```python
from build123d import *

# Parameters (mm, degrees)
SKETCH1_R           = 13.45
BOSS_EXTRUDE2_DEPTH = 48
SKETCH7_W           = 44
SKETCH7_H           = 14
SKETCH7_R           = 4.25
SKETCH7_R_2         = 4.1
BOSS_EXTRUDE3_DEPTH = 13
FILLET1_R           = 3
FILLET2_R           = 5
FILLET3_R           = 5
FILLET4_R           = 3


with BuildPart() as part:
    # Sketch1 → Boss-Extrude2 (new body)
    with BuildSketch(Plane(origin=(0, 0, 0), x_dir=(1, 0, 0), z_dir=(0, 1, 0))):
        Polygon((-17.4, 17.4), (17.4, 17.4), (17.4, -17.4), (-17.4, -17.4), (-17.4, 13.4), (-82.6, 13.4), (-82.6, 17.4), align=None)
        with Locations(Location((0, 0, 0), (0, 0, 270))):
            Circle(SKETCH1_R, mode=Mode.SUBTRACT)
    boss_extrude2 = extrude(amount=BOSS_EXTRUDE2_DEPTH)

    # Mirror2: Boss-Extrude2 across plane
    add(boss_extrude2.mirror(Plane(origin=(-82.6, 48, -17.4), x_dir=(0, 0, 1), z_dir=(1, 0, 0))))

    # Sketch7 → Boss-Extrude3 (add)
    with BuildSketch(Plane.XY.offset(-13.4)):
        with Locations((-97.6, 24)):
            Rectangle(SKETCH7_W, SKETCH7_H)
        with Locations(Location((-82.6, 24, 0), (0, 0, 180))):
            Circle(SKETCH7_R, mode=Mode.SUBTRACT)
        with Locations(Location((-112.6, 24, 0), (0, 0, 180))):
            Circle(SKETCH7_R_2, mode=Mode.SUBTRACT)
    extrude(amount=BOSS_EXTRUDE3_DEPTH)

    # Fillet1
    fillet1_edges = [part.edges().sort_by_distance(p)[0] for p in [
        (17.4, 24, 17.4),
        (-17.4, 24, 17.4),
        (-182.6, 24, 17.4),
        (-147.8, 24, 17.4),
    ]]
    fillet(fillet1_edges, radius=FILLET1_R)

    # Fillet2
    fillet2_edges = [part.edges().sort_by_distance(p)[0] for p in [
        (-17.4, 24, -13.4),
        (17.4, 24, -17.4),
        (-182.6, 24, -17.4),
        (-147.8, 24, -13.4),
    ]]
    fillet(fillet2_edges, radius=FILLET2_R)

    # Fillet3
    fillet3_edges = [part.edges().sort_by_distance(p)[0] for p in [
        (-75.6, 17, -6.9),
        (-75.6, 31, -6.9),
        (-119.6, 31, -6.9),
        (-119.6, 17, -6.9),
    ]]
    fillet(fillet3_edges, radius=FILLET3_R)

    # Fillet4
    fillet4_edges = [part.edges().sort_by_distance(p)[0] for p in [
        (-97.6, 31, -13.4),
        (-75.6, 24, -13.4),
        (-97.6, 17, -13.4),
        (-119.6, 24, -13.4),
        (-77.064466094, 29.535533906, -13.4),
        (-77.064466094, 18.464466094, -13.4),
        (-118.135533906, 29.535533906, -13.4),
        (-118.135533906, 18.464466094, -13.4),
    ]]
    fillet(fillet4_edges, radius=FILLET4_R)


solid = part.part
```
Geometry: final body of the model. Coordinates: model frame, mm. A direction names the side the tool comes from. Give positions to 0.01 mm unless a question says otherwise; leave off trailing zeros. Loops run counter-clockwise (first coordinate to the right, second up) from the corner with the lowest first, then second, coordinate; pieces in that order, holes last. Notation, with made-up numbers: (20, 75.5) - (66, 75.5) arc R23 cw to (66, 87.5) - close; hole circle Ø9 at (8.25, 5.5). An arc over 180 degrees is marked (long way). Answer as CSV lines item,"result". Start each with the question number.
(1) Reachability of faces 4 (the face through (-98, 31, -5)), 5 (the face through (-17.4, 24, 3)), 6 (the face through (-118.17, 18.5, -5.33)) from +Z, -Z, +X, -X, +Y, -Y: full face, straight path, thin tool, end or side. Return the list, or none.
(2) Pin query (flat end, axial travel): P1, Ø15.5, axis at x = -102.5, y = 25, coming from the +Z side; P2, Ø11, axis at x = -103.5, z = -3, coming from the +Y side; P3, Ø16, axis at x = -165.2, z = 0, coming from the +Y side; P4, Ø3, axis at y = 14.5, z = -13.5, coming from the -X side. Return the tip coordinate at first contact, or that it passes through.
(3) Ray query, line 1 along X through (y, z) = (22.5, 0); line 2 along Y through (x, z) = (-112.6, -5.25); line 3 along Y through (x, z) = (-82.6, -4.75). Return the intervals inside material, ascending. Write a range as [from, to].
(4) Mould query, pull axis X, two halves, no side actions, for faces 1 (the face through (-181.17, 24.34, -15.9)), 2 (the face through (-18.9, 24.34, -11.97)), 3 (the face through (-165, 24, 17.4)). Classes: +X half, -X half, draft (parallel to the pull), parting line (faces both ways), or undercut.
(5) Section query B-B (z = -3). Output: boundary loops of the cut face in (x, y).
(6) Section query C-C (y = 24). Give the number of separate pieces and of enclosed holes in the cut face, and give its area (3 significant figures).
(7) Section query D-D (z = 11.5). Output: boundary loops of the cut face in (x, y).
(8) Section query A-A (x = 0). Output: boundary loops of the cut face in (y, z), and give its area (3 significant figures).
Worked answers:
1,face 4,"+Z, +Y"
1,face 5,"+Z, +Y, -Y"
1,face 6,"+Z, -Y"
2,P1,"stops at z = -0.4"
2,P2,"stops at y = 31"
2,P3,"passes through"
2,P4,"stops at x = -182.6"
3,line 1,"x = [-182.6, -178.65], [-151.75, -147.8], [-17.4, -13.45], [13.45, 17.4]"
3,line 2,"y = [17, 19.9], [28.1, 31]"
3,line 3,"y = [17, 19.75], [28.25, 31]"
4,face 1,"-X half"
4,face 2,"undercut"
4,face 3,"draft"
5,outline,"(-182.6, 0) - (-178.31, 0) - (-178.31, 48) - (-182.6, 48) - close; (-152.09, 0) - (-147.8, 0) - (-147.8, 48) - (-152.09, 48) - close; (-119.6, 22) arc R5 ccw to (-114.6, 17) - (-80.6, 17) arc R5 ccw to (-75.6, 22) - (-75.6, 26) arc R5 ccw to (-80.6, 31) - (-114.6, 31) arc R5 ccw to (-119.6, 26) - close; (-17.4, 0) - (-13.11, 0) - (-13.11, 48) - (-17.4, 48) - close; (13.11, 0) - (17.4, 0) - (17.4, 48) - (13.11, 48) - close; hole circle Ø8.2 at (-112.6, 24); hole circle Ø8.5 at (-82.6, 24)"
6,separate pieces,"1"
6,enclosed holes,"2"
6,area,"2,160 mm^2"
7,outline,"(-182.6, 0) - (-172.18, 0) - (-172.18, 48) - (-182.6, 48) - close; (-158.22, 0) - (-147.8, 0) - (-147.8, 48) - (-158.22, 48) - close; (-17.4, 0) - (-6.98, 0) - (-6.98, 48) - (-17.4, 48) - close; (6.98, 0) - (17.4, 0) - (17.4, 48) - (6.98, 48) - close"
8,outline,"(0, -17.4) - (48, -17.4) - (48, -13.45) - (0, -13.45) - close; (0, 13.45) - (48, 13.45) - (48, 17.4) - (0, 17.4) - close"
8,area,"379 mm^2"
